Check sheet for the modelled part. Datum: model origin and axes. Units: mm. Face numbers are marked on the shaded views. Give positions to 0.01 mm unless a question says otherwise; leave off trailing zeros. Order: outer loops, then holes, each group sorted by start corner. A loop starts at its lowest first (then second) coordinate and runs counter-clockwise, first axis right, second up.
from build123d import *

# Parameters (mm, degrees)
ESQUISSE1_R        = 1.6
ESQUISSE1_R_2      = 3
BOSS_EXTRU_1_DEPTH = 1


with BuildPart() as part:
    # Esquisse1 → Boss.-Extru.1 (new body)
    with BuildSketch(Plane.XY):
        with BuildLine():
            ThreePointArc((33.844669118, -3.246285927), (30.75, 0), (33.844669118, 3.246285927))
            ThreePointArc((33.844669118, 3.246285927), (29.444863729, 17), (19.733700639, 27.687200275))
            ThreePointArc((19.733700639, 27.687200275), (15.375, 26.630281166), (14.110968478, 30.933486202))
            ThreePointArc((14.110968478, 30.933486202), (0, 34), (-14.110968478, 30.933486202))
            ThreePointArc((-14.110968478, 30.933486202), (-13.841531032, 30.210744775), (-13.75, 29.444863729))
            ThreePointArc((-13.75, 29.444863729), (-16.084037959, 26.326608842), (-19.733700639, 27.687200275))
            ThreePointArc((-19.733700639, 27.687200275), (-29.444863729, 17), (-33.844669118, 3.246285927))
            ThreePointArc((-33.844669118, 3.246285927), (-31.64762616, 2.242506927), (-30.75, 0))
            ThreePointArc((-30.75, 0), (-31.64762616, -2.242506927), (-33.844669118, -3.246285927))
            ThreePointArc((-33.844669118, -3.246285927), (-29.444863729, -17), (-19.733700639, -27.687200275))
            ThreePointArc((-19.733700639, -27.687200275), (-16.084037959, -26.326608842), (-13.75, -29.444863729))
            ThreePointArc((-13.75, -29.444863729), (-13.841531032, -30.210744775), (-14.110968478, -30.933486202))
            ThreePointArc((-14.110968478, -30.933486202), (0, -34), (14.110968478, -30.933486202))
            ThreePointArc((14.110968478, -30.933486202), (15.375, -26.630281166), (19.733700639, -27.687200275))
            ThreePointArc((19.733700639, -27.687200275), (29.444863729, -17), (33.844669118, -3.246285927))
        make_face()
        with Locations((-15.5, -15.5)):
            Circle(ESQUISSE1_R, mode=Mode.SUBTRACT)
        with Locations((15.5, -15.5)):
            Circle(ESQUISSE1_R, mode=Mode.SUBTRACT)
        with Locations((-15.5, 15.5)):
            Circle(ESQUISSE1_R, mode=Mode.SUBTRACT)
        Circle(ESQUISSE1_R_2, mode=Mode.SUBTRACT)
        with Locations((15.5, 15.5)):
            Circle(ESQUISSE1_R, mode=Mode.SUBTRACT)
    extrude(amount=BOSS_EXTRU_1_DEPTH)


solid = part.part
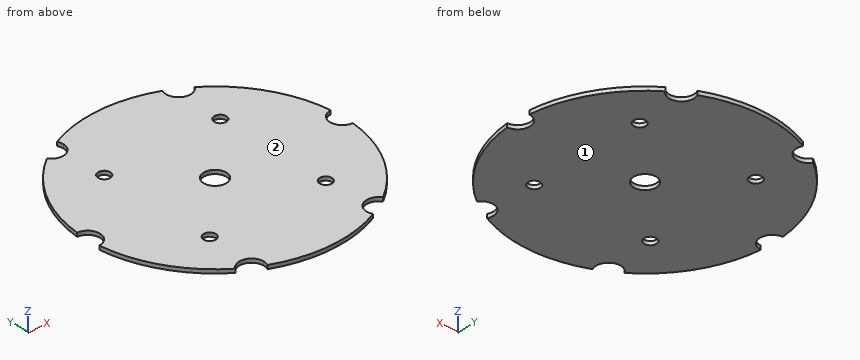
1) Material ranges on L1, parallel to Y at x = 15.5, z = 0.75; L2, parallel to Y at x = 0, z = 0.6; L3, parallel to X at y = -26, z = 0.2, recorded low to high.
Recorded:
L1: y = -26.56 to -17.1, -13.9 to 13.9, 17.1 to 26.56
L2: y = -34 to -3, 3 to 34
L3: x = -21.91 to 21.91
2) Section check A-A, the plane z = 0.4. Record the cut outline in (x, y).
Recorded:
outline: (-33.84, -3.25) arc R34 ccw to (-19.73, -27.69) arc R3.25 cw to (-14.11, -30.93) arc R34 ccw to (14.11, -30.93) arc R3.25 cw to (19.73, -27.69) arc R34 ccw to (33.84, -3.25) arc R3.25 cw to (33.84, 3.25) arc R34 ccw to (19.73, 27.69) arc R3.25 cw to (14.11, 30.93) arc R34 ccw to (-14.11, 30.93) arc R3.25 cw to (-19.73, 27.69) arc R34 ccw to (-33.84, 3.25) arc R3.25 cw to start; hole circle Ø3.2 at (-15.5, -15.5); hole circle Ø3.2 at (-15.5, 15.5); hole circle Ø6 at (0, 0); hole circle Ø3.2 at (15.5, -15.5); hole circle Ø3.2 at (15.5, 15.5)
3) Depth check by flat-ended pin: pin 1 Ø1.9 at (x, y) = (15.5, 15.5) entering from +Z. Enter the tip coordinate at first touch or a pass-through.
Recorded:
pin 1: passes through
4) Draft check along Z on the marked faces 1 and 2. Enter one of: +Z half, -Z half, draft (parallel to the pull), parting line (faces both ways), or undercut.
Recorded:
face 1: -Z half
face 2: +Z half
5) Section check B-B, the plane y = -15.5. Record the cut outline in (x, z), then the cut area to 3 significant figures.
Recorded:
outline: (-30.26, 0) - (-17.1, 0) - (-17.1, 1) - (-30.26, 1) - close; (-13.9, 0) - (13.9, 0) - (13.9, 1) - (-13.9, 1) - close; (17.1, 0) - (30.26, 0) - (30.26, 1) - (17.1, 1) - close
area: 54.1 mm2
6) Section check D-D, the plane x = 15.5. Record the cut outline in (y, z).
Recorded:
outline: (-26.56, 0) - (-17.1, 0) - (-17.1, 1) - (-26.56, 1) - close; (-13.9, 0) - (13.9, 0) - (13.9, 1) - (-13.9, 1) - close; (17.1, 0) - (26.56, 0) - (26.56, 1) - (17.1, 1) - close
7) Section check C-C, the plane x = -1. Record the cut outline in (y, z).
Recorded:
outline: (-33.99, 0) - (-2.83, 0) - (-2.83, 1) - (-33.99, 1) - close; (2.83, 0) - (33.99, 0) - (33.99, 1) - (2.83, 1) - close
